Answer from the drawing. Dimensions are ordinates in mm from the lowest x, y and z of the part. A direction names the side the tool comes from. Give positions to 0.01 mm unless a question says otherwise; leave off trailing zeros. Loops run counter-clockwise (first coordinate to the right, second up) from the corner with the lowest first, then second, coordinate; pieces in that order, holes last.
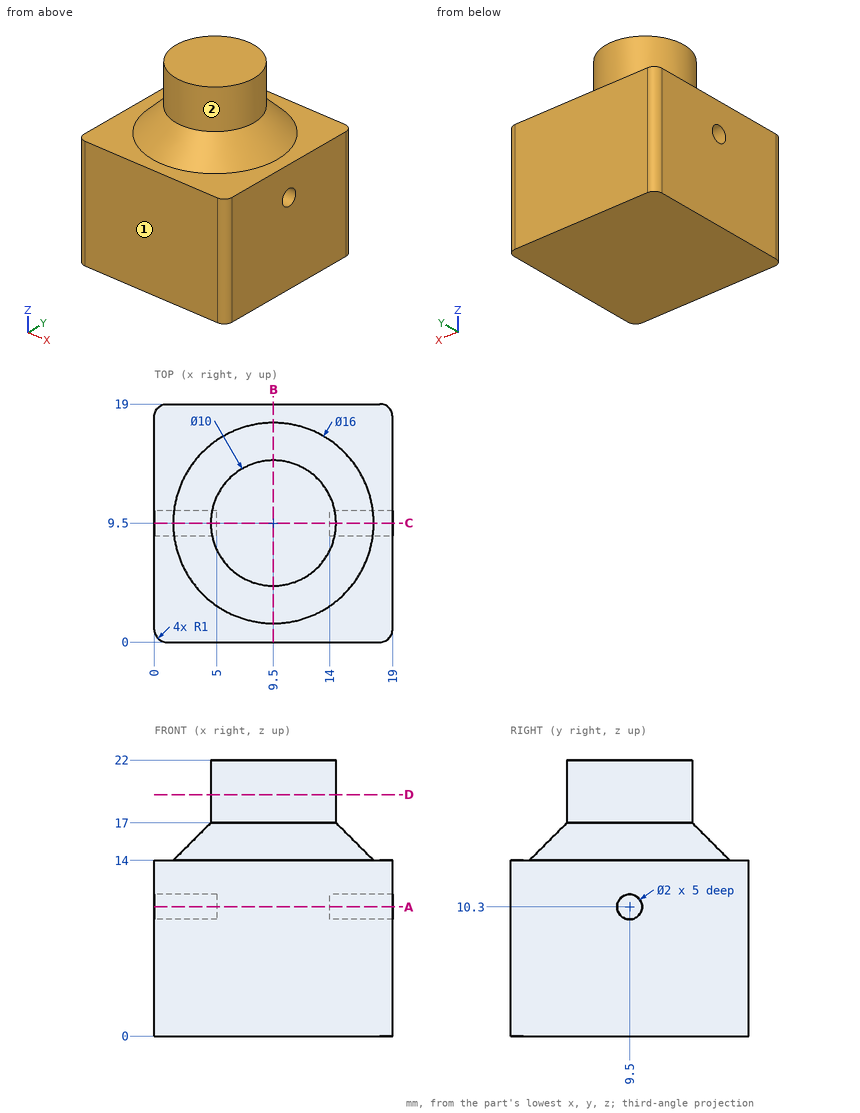
Item 1: Consider line 1 (Y direction, x = 15.4, z = 10.3); line 2 (Z direction, x = 17.5, y = 2.25); line 3 (Z direction, x = 1.55, y = 9.5). Determine where each line is inside the solid, lowest interval first.
Item 2: Find section A-A, the plane z = 10.3. Write down the section's boundary in (x, y).
Item 3: For the marked faces 1 and 2, determine the directions among +Z, -Z, +X, -X, +Y, -Y from which every point of the face is accessible in a straight line to the end or side of a thin tool.
Item 4: Find section B-B, the plane x = 9.5. Write down the section's boundary in (y, z), plus the area to 3 significant figures.
Item 5: Find section C-C, the plane y = 9.5. Write down the section's boundary in (x, z).
Item 6: Find section D-D, the plane z = 19.25. Write down the section's boundary in (x, y).
Item 7: Flat-ended cylindrical pins translate along their axes: pin 1 Ø1.5 at (y, z) = (13.5, 15) entering from +X; pin 2 Ø2 at (x, z) = (7, 19.5) entering from +Y. Find the tip coordinate at first contact, or state that the pin passes through.
Ans:
1. line 1: y = 0 to 8.5, 10.5 to 19
1. line 2: z = 0 to 14
1. line 3: z = 0 to 9.3, 11.3 to 14.05
2. outline: (0, 1) arc R1 ccw to (1, 0) - (18, 0) arc R1 ccw to (19, 1) - (19, 8.5) - (14, 8.5) - (14, 10.5) - (19, 10.5) - (19, 18) arc R1 ccw to (18, 19) - (1, 19) arc R1 ccw to (0, 18) - (0, 10.5) - (5, 10.5) - (5, 8.5) - (0, 8.5) - close
3. face 1: +Z, -Z, +X, -X, -Y
3. face 2: +Z
4. outline: (0, 0) - (19, 0) - (19, 14) - (17.5, 14) - (14.5, 17) - (14.5, 22) - (4.5, 22) - (4.5, 17) - (1.5, 14) - (0, 14) - close
4. area: 355 mm2
5. outline: (0, 0) - (19, 0) - (19, 9.3) - (14, 9.3) - (14, 11.3) - (19, 11.3) - (19, 14) - (17.5, 14) - (14.5, 17) - (14.5, 22) - (4.5, 22) - (4.5, 17) - (1.5, 14) - (0, 14) - (0, 11.3) - (5, 11.3) - (5, 9.3) - (0, 9.3) - close
6. outline: circle Ø10 at (9.5, 9.5)
7. pin 1: stops at x = 16.24
7. pin 2: stops at y = 14.27
